Model file for the job. Use its own axes, mm. Face numbers are marked on the shaded views. A direction names the side the tool comes from. Round coordinates to 2 decimals unless told otherwise and drop trailing zeros. Loops run counter-clockwise (first coordinate to the right, second up) from the corner with the lowest first, then second, coordinate; pieces in that order, holes last. Notation, with made-up numbers: (88, 83.5) - (116, 83.5) arc R37 ccw to (116, 119.5) - close; hole circle Ø5 at (-27, 11.5). An arc over 180 degrees is marked (long way). Use one line per item in the form item = value.
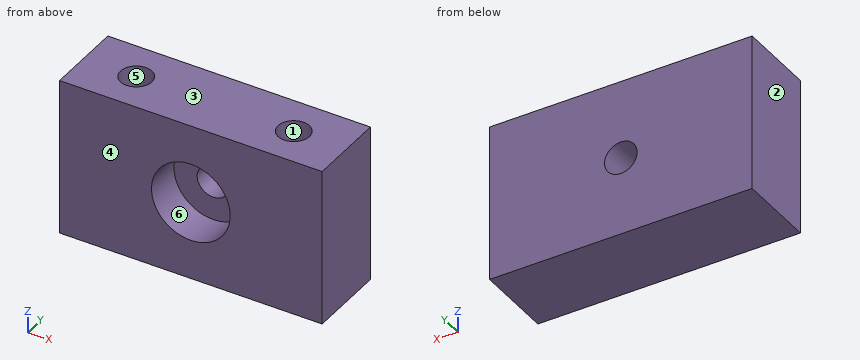
from build123d import *

# Parameters (mm, degrees)
F0_W     = 50
F0_H     = 30
F0_R     = 7.5
F1_DEPTH = 15
F0_R_2   = 3.1
F2_DEPTH = 8
F3_R     = 3
F4_DEPTH = 20


with BuildPart() as f1:
    # F0 (on Front) → F1 (new body)
    with BuildSketch(Plane.XZ):
        Rectangle(F0_W, F0_H)
        Circle(F0_R, mode=Mode.SUBTRACT)
    extrude(amount=F1_DEPTH)

    # F0 (on Front) → F2 (join)
    with BuildSketch(Plane.XZ):
        Circle(F0_R)
        Circle(F0_R_2, mode=Mode.SUBTRACT)
    extrude(amount=F2_DEPTH)

    # F3 (on face) → F4 (cut)
    with BuildSketch(Plane.XY.offset(15)):
        with Locations((-15, -7.5)):
            Circle(F3_R)
        with Locations((15, -7.5)):
            Circle(F3_R)
    extrude(amount=-F4_DEPTH, mode=Mode.SUBTRACT)


solid = f1.part
1. Flat gauge pins, fed straight in: pin 1 (3 mm diameter, centred on x = -15, y = -8.5, fed in from +Z); pin 2 (7 mm diameter, centred on x = 0, z = 0, fed in from -Y). Where does each tip first touch, or does it go through?
Geometry check:
pin_1 = -5
pin_2 = -8
2. Cut at B-B, the plane x = 15. Give the cut face in (y, z).
Geometry check:
outline = (-15, -15) - (0, -15) - (0, 15) - (-4.5, 15) - (-4.5, -5) - (-10.5, -5) - (-10.5, 15) - (-15, 15) - close
3. Wall check: probe 1 along Y at (x, z) = (-15, 10.25); probe 2 along Z at (x, y) = (0, -4); probe 3 along X at (y, z) = (-5.5, -1.5). Give the ranges that are in metal, low to high.
Geometry check:
probe_1 = -15 to -10.5, -4.5 to 0
probe_2 = -15 to -3.1, 3.1 to 15
probe_3 = -25 to -17.24, -12.76 to -2.71, 2.71 to 12.76, 17.24 to 25
4. Pull direction X, two halves, no side cores. Call the marked faces 1, 2 and 3: +X half, -X half, draft (parallel to the pull), parting line (faces both ways), or undercut.
Geometry check:
face_1 = undercut
face_2 = -X half
face_3 = draft
5. Tool access for the marked faces 4, 5 and 6: list every direction of +Z, -Z, +X, -X, +Y, -Y with a clear straight run to the whole face (end or side of a thin tool).
Geometry check:
face_4 = +Z, -Z, +X, -X, -Y
face_5 = +Z
face_6 = -Y
6. Cut at C-C, the plane y = -7.5. Give the cut face in (x, z).
Geometry check:
outline = (-25, -15) - (25, -15) - (25, 15) - (18, 15) - (18, -5) - (12, -5) - (12, 15) - (-12, 15) - (-12, -5) - (-18, -5) - (-18, 15) - (-25, 15) - close; hole circle Ø6.2 at (0, 0)
7. Cut at D-D, the plane x = 6.5. Give the cut face in (y, z).
Geometry check:
outline = (-15, -15) - (0, -15) - (0, 15) - (-15, 15) - (-15, 3.74) - (-8, 3.74) - (-8, -3.74) - (-15, -3.74) - close
8. Cut at A-A, the plane y = -12.5. Give the cut face in (x, z), plus the area to 3 significant figures.
Geometry check:
outline = (-25, -15) - (25, -15) - (25, 15) - (-25, 15) - close; hole circle Ø15 at (0, 0)
area = 1,320 mm^2
